from build123d import *

# Parameters (mm, degrees)
F1_DEPTH = 10
F3_D     = 4
F3_DEPTH = 12
F3_TIP   = 1.2017212381


# Not quite as in the source:
# - a feature names something its author has since deleted; it is built from what else it names


with BuildPart() as f1:
    # F0 (on Right) → F1 (new body)
    with BuildSketch(Plane.YZ):
        Polygon((22.9933855712, -5), (22.9933855712, 5), (-4.6191914314, 5), (22.9933855712, 64.2153624752), (13.9303077009, 68.4415450926), (-15.652970621, 5), (-31.6901920953, 5), (-31.8974178605, 15), (-41.8974178605, 15), (-41.8974178605, -5), align=None)
    extrude(amount=F1_DEPTH)

    # F3
    with Locations(Plane.YZ.offset(10)):
        with Locations((16.3487553273, 61.7969148487), (17.9933855712, 0), (-9.4260048308, 0), (-36.8453457878, 0.0520720727), (3.1063371506, 33.3984574243), (-36.8456114192, 9.9481935587)):
            Hole(F3_D / 2, depth=F3_DEPTH)
            with Locations((0, 0, -(F3_DEPTH + F3_TIP / 2))):  # 118° drill point
                Cone(0, F3_D / 2, F3_TIP, mode=Mode.SUBTRACT)


solid = f1.part
Verification items for the finished model (mm, model axes). A direction names the side the tool comes from. Give positions to 0.01 mm unless a question says otherwise; leave off trailing zeros. Write each loop counter-clockwise with the first axis right and the second up, starting at its lowest first coordinate (ties: lowest second). Pieces come first, ordered by that corner, then holes. Notation, with made-up numbers: M 57.25,1 L 84.25,1 A25 cw 84.25,32 Z; hole C 73.25,89.5 d8. An arc over 180 degrees is marked long. Put each result on its own line as item: value. Start each with the question number.
1. Section check D-D (y = -21). Record the cut outline in (x, z), and give its area (3 significant figures).
2. Section check A-A (y = 6.5). Record the cut outline in (x, z), and give its area (3 significant figures).
3. Scan lines: line 1 along Z through (x, y) = (5.5, -36.5); line 2 along Z through (x, y) = (1, 4.5); line 3 along Z through (x, y) = (4.5, 18). Record each from-to range of solid material in increasing order. Write a range as [from, to].
4. Section check C-C (x = 3). Record the cut outline in (y, z), and give its area (3 significant figures).
5. Draft check along Z on faces 1 (the face through (0, -5, 16)), 2 (the face through (4.93, -0.654, 37.165)), 3 (the face through (4.93, 2.183, 31.624)). Enter one of: +Z half, -Z half, draft (parallel to the pull), parting line (faces both ways), or undercut.
6. Go/stop test with flat-tipped pins: pin 1 Ø1 at (x, z) = (2.5, 57) entering from +Y; pin 2 Ø5 at (x, y) = (7, -27.5) entering from +Z; pin 3 Ø1.5 at (x, z) = (3.5, 32.5) entering from +Y. Record where each tip stops, or that it passes through.
7. Set-up check for faces 4 (the face through (4.93, -34.848, 10.036)), 5 (the face through (4.93, 8.994, 34.193)), 6 (the face through (5, -37, 15)), 7 (the face through (5, -24, 5)): record each of +Z, -Z, +X, -X, +Y, -Y from which the full face is reachable in a straight line by a thin tool's end or side.
8. Section check B-B (z = 7). Record the cut outline in (x, y), and give its area (3 significant figures).
Answer list:
1. outline: M 0,-5 L 10,-5 L 10,5 L 0,5 Z
1. area: 100 mm2
2. outline: M 0,-5 L 10,-5 L 10,5 L 0,5 Z; M 0,28.85 L 10,28.85 L 10,52.51 L 0,52.51 Z
2. area: 337 mm2
3. line 1: [-5, -1.92], [2.02, 7.98], [11.92, 15]
3. line 2: [-5, 5], [24.56, 31.96], [34.83, 48.22]
3. line 3: [-5, -2], [2, 5], [53.51, 60.67], [62.93, 66.54]
4. outline: M -41.9,-5 L 22.99,-5 L 22.99,5 L -4.62,5 L 22.99,64.22 L 13.93,68.44 L -15.65,5 L -31.69,5 L -31.9,15 L -41.9,15 Z; hole C -36.85,0.05 d4; hole C -36.85,9.95 d4; hole C -9.43,0 d4; hole C 3.11,33.4 d4; hole C 16.35,61.8 d4; hole C 17.99,0 d4
4. area: 1,350 mm2
5. face 1: draft
5. face 2: +Z half
5. face 3: undercut
6. pin 1: y = 19.86
6. pin 2: z = 5
6. pin 3: y = 8.55
7. face 4: +X, -X
7. face 5: +X, -X, +Y
7. face 6: +Z, +X, -X, -Y
7. face 7: +Z, +X, -X
8. outline: M 0,-41.9 L 10,-41.9 L 10,-31.73 L 0,-31.73 Z; M 0,-14.72 L 10,-14.72 L 10,-3.69 L 0,-3.69 Z
8. area: 212 mm2
